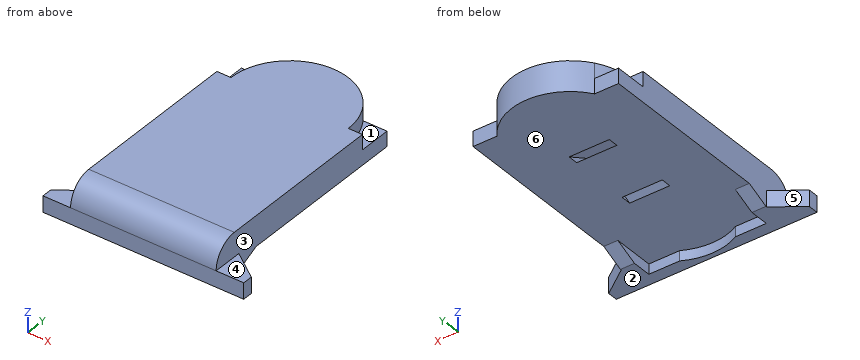
from build123d import *

# Parameters (mm, degrees)
PAD_DEPTH            = 4
POCKET_DEPTH         = 1.5
POCKET004_DEPTH      = 2.4
POCKET005_DEPTH      = 10.001
POCKET005_DEPTH_BACK = -10.001
POCKET006_DEPTH      = 10.001
POCKET006_DEPTH_BACK = -10.001
POCKET007_DEPTH      = 1
POCKET008_DEPTH      = 2


with BuildPart() as part:
    # Sketch → Pad (new body)
    with BuildSketch(Plane.XY):
        with BuildLine():
            Line((-10, 0), (10, 0))
            Line((10, 0), (10, 1))
            Line((10, 1), (7.25, 3))
            Line((7.25, 3), (7.25, 22.6))
            Line((7.25, 22.6), (4.864155, 22.6))
            ThreePointArc((4.864155, 22.6), (0, 25.2), (-4.864155, 22.6))
            Line((-7.25, 22.6), (-4.864155, 22.6))
            Line((-7.25, 3), (-7.25, 22.6))
            Line((-10, 1), (-7.25, 3))
            Line((-10, 0), (-10, 1))
        make_face()
    extrude(amount=PAD_DEPTH)

    # Sketch001 (on Face12 of Pad) → Pocket (cut)
    with BuildSketch(Plane.XY.offset(4)):
        with BuildLine():
            ThreePointArc((-4.864155, 22.6), (-5.598116, 21.048116), (-5.85, 19.35))
            Line((-5.85, 19.35), (-7.25, 19.35))
            Line((-7.25, 19.35), (-7.25, 22.6))
            Line((-4.864155, 22.6), (-7.25, 22.6))
        make_face()
        with BuildLine():
            ThreePointArc((5.85, 19.35), (5.598116, 21.048116), (4.864155, 22.6))
            Line((7.25, 22.6), (4.864155, 22.6))
            Line((7.25, 19.35), (7.25, 22.6))
            Line((5.85, 19.35), (7.25, 19.35))
        make_face()
    extrude(amount=-POCKET_DEPTH, mode=Mode.SUBTRACT)

    # Sketch005 (on Face12 of Pad) → Pocket004 (cut)
    with BuildSketch(Plane.XY.offset(4)):
        Polygon((-7.25, 3), (-10, 1), (-10, 0), (-7.25, 0), align=None)
        Polygon((7.25, 3), (10, 1), (10, 0), (7.25, 0), align=None)
    extrude(amount=-POCKET004_DEPTH, mode=Mode.SUBTRACT)

    # Sketch006 → Pocket005 (cut, two sides)
    with BuildSketch(Plane.YZ) as pocket005_sk:
        with BuildLine():
            ThreePointArc((2.4, 4), (0.702944, 3.297056), (0, 1.6))
            Line((0, 1.6), (0, 4))
            Line((2.4, 4), (0, 4))
        make_face()
    extrude(amount=-POCKET005_DEPTH, mode=Mode.SUBTRACT)
    extrude(pocket005_sk.sketch, amount=-POCKET005_DEPTH_BACK, mode=Mode.SUBTRACT)

    # Sketch007 → Pocket006 (cut, two sides)
    with BuildSketch(Plane.YZ) as pocket006_sk:
        Polygon((3.1, 0), (5.3, 1), (25.2, 1), (25.2, 0), align=None)
    extrude(amount=-POCKET006_DEPTH, mode=Mode.SUBTRACT)
    extrude(pocket006_sk.sketch, amount=-POCKET006_DEPTH_BACK, mode=Mode.SUBTRACT)

    # Sketch008 → Pocket007 (cut)
    with BuildSketch(Plane.XY):
        with BuildLine():
            Line((-5.85, 5.3), (-5.85, 1.2))
            Line((-5.85, 1.2), (-2.774887, 1.2))
            ThreePointArc((-2.774887, 1.2), (0, 0.5), (2.774887, 1.2))
            Line((5.85, 1.2), (2.774887, 1.2))
            Line((5.85, 5.3), (5.85, 1.2))
            Line((-5.85, 5.3), (5.85, 5.3))
        make_face()
    extrude(amount=POCKET007_DEPTH, mode=Mode.SUBTRACT)

    # Sketch009 → Pocket008 (cut, symmetric)
    with BuildSketch(Plane.YZ):
        Polygon((8.85, 1), (11.85, 2.5), (13.85, 2.5), (16.85, 1), (15.85, 1), (13.35, 1.5), (12.35, 1.5), (9.85, 1), align=None)
    extrude(amount=POCKET008_DEPTH, both=True, mode=Mode.SUBTRACT)


solid = part.part
The listing builds one solid part. Answer for the finished solid, in the listing's coordinates (mm). Face numbers are marked on the shaded views. A direction names the side the tool comes from. Coordinates: 2 decimals unless noted, no trailing zeros. Order: outer loops, then holes, each group sorted by start corner. A loop starts at its lowest first (then second) coordinate and runs counter-clockwise, first axis right, second up.
Q1. A cutting plane is placed at B-B, the plane x = 0.5. Write down the section's boundary in (y, z).
Q2. Given P1, Ø1.6, axis at y = 12.5, z = 1.5, coming from the -X side; P2, Ø1.5, axis at x = -1.5, y = 14.5, coming from the -Z side; P3, Ø0.8, axis at y = 14, z = 1.5, coming from the +X side, each flat-ended and moving along its own axis, determine where each tip first touches the part or whether it passes through.
Q3. Consider line 1 (X direction, y = 14, z = 1.5); line 2 (Z direction, x = -1.25, y = 21); line 3 (X direction, y = 18, z = 3.55). Determine where each line is inside the solid, lowest interval first.
Q4. For a pull along X with two mould halves and no side action, classify the marked faces 3, 4, 5 and 6 as pulls with the +X half, pulls with the -X half, needs draft (parallel to the pull), parting line crosses it, or undercut.
Q5. Which of the six approach directions +Z, -Z, +X, -X, +Y, -Y give full straight-line access (tool end or side, diameter ignored) to the marked faces 1 and 2?
Q6. A cutting plane is placed at D-D, the plane z = 1.9. Write down the section's boundary in (x, y), and give its area (3 significant figures).
Q7. A cutting plane is placed at A-A, the plane y = 11.25. Write down the section's boundary in (x, z), and give its area (3 significant figures).
Q8. A cutting plane is placed at C-C, the plane z = 3.2. Write down the section's boundary in (x, y), and give its area (3 significant figures).
Answers follow:
1. outline: (0, 0) - (0.52, 0) - (0.52, 1) - (8.85, 1) - (11.85, 2.5) - (13.85, 2.5) - (16.85, 1) - (25.18, 1) - (25.18, 4) - (2.4, 4) arc R2.4 ccw to (0, 1.6) - close; (9.85, 1) - (15.85, 1) - (13.35, 1.5) - (12.35, 1.5) - close
2. P1: stops at x = -7.25
2. P2: stops at z = 1
2. P3: stops at x = 7.25
3. line 1: x = -7.25 to -2, 2 to 7.25
3. line 2: z = 1 to 4
3. line 3: x = -7.25 to 7.25
4. face 3: pulls with the +X half
4. face 4: needs draft
4. face 5: pulls with the -X half
4. face 6: undercut
5. face 1: +Z, +X, +Y
5. face 2: -Z, +X, -X, +Y, -Y
6. outline: (-7.25, 0.02) - (7.25, 0.02) - (7.25, 22.6) - (4.86, 22.6) arc R5.85 ccw to (-4.86, 22.6) - (-7.25, 22.6) - close; hole (-2, 10.65) - (2, 10.65) - (2, 15.05) - (-2, 15.05) - close
6. area: 328 mm2
7. outline: (-7.25, 1) - (7.25, 1) - (7.25, 4) - (-7.25, 4) - close; hole (-2, 1.28) - (2, 1.28) - (2, 2.2) - (-2, 2.2) - close
7. area: 39.8 mm2
8. outline: (-7.25, 0.61) - (7.25, 0.61) - (7.25, 19.35) - (5.85, 19.35) arc R5.85 ccw to (4.86, 22.6) arc R5.85 ccw to (-4.86, 22.6) arc R5.85 ccw to (-5.85, 19.35) - (-7.25, 19.35) - close
8. area: 325 mm2
